from build123d import *

# Parameters (mm, degrees)
SCHIZZO1_R                   = 2.1
ESTRUSIONE_ESTRUSIONE1_DEPTH = 4
SCHIZZO2_R                   = 2.5
TAGLIO_ESTRUSIONE1_DEPTH     = 4
SCHIZZO3_R                   = 1.5
TAGLIO_ESTRUSIONE3_DEPTH     = 4


with BuildPart() as part:
    # Schizzo1 → Estrusione-Estrusione1 (new body)
    with BuildSketch(Plane.XY):
        with BuildLine():
            Line((69.543022759, -257.170330876), (65.21289574, -264.670330876))
            ThreePointArc((65.21289574, -264.670330876), (57.892387664, -271.990838952), (47.892387664, -274.670330876))
            Line((47.892387664, -274.670330876), (20.986398432, -274.670330876))
            ThreePointArc((20.986398432, -274.670330876), (10.986398432, -271.990838952), (3.665890356, -264.670330876))
            Line((3.665890356, -264.670330876), (-0.664236663, -257.170330876))
            Line((-0.664236663, -257.170330876), (-250.664236663, 175.842371016))
            Line((-250.664236663, 175.842371016), (-254.994363682, 183.342371016))
            ThreePointArc((-254.994363682, 183.342371016), (-257.673855606, 193.342371016), (-254.994363682, 203.342371016))
            Line((-254.994363682, 203.342371016), (-241.541369065, 226.643641206))
            ThreePointArc((-241.541369065, 226.643641206), (-234.22086099, 233.964149281), (-224.22086099, 236.643641206))
            Line((-224.22086099, 236.643641206), (-215.560606952, 236.643641206))
            Line((-215.560606952, 236.643641206), (284.439393048, 236.643641206))
            Line((284.439393048, 236.643641206), (293.099647086, 236.643641206))
            ThreePointArc((293.099647086, 236.643641206), (303.099647086, 233.964149281), (310.420155162, 226.643641206))
            Line((310.420155162, 226.643641206), (323.873149778, 203.342371016))
            ThreePointArc((323.873149778, 203.342371016), (326.552641702, 193.342371016), (323.873149778, 183.342371016))
            Line((323.873149778, 183.342371016), (319.543022759, 175.842371016))
            Line((319.543022759, 175.842371016), (69.543022759, -257.170330876))
        make_face()
        with Locations((34.439393048, -259.670330876)):
            Circle(SCHIZZO1_R, mode=Mode.SUBTRACT)
        with Locations((304.156271413, 207.493006111)):
            Circle(SCHIZZO1_R, mode=Mode.SUBTRACT)
        with Locations((-235.277485317, 207.493006111)):
            Circle(SCHIZZO1_R, mode=Mode.SUBTRACT)
    extrude(amount=ESTRUSIONE_ESTRUSIONE1_DEPTH)

    # Schizzo2 → Taglio-Estrusione1 (cut)
    with BuildSketch(Plane.XY.offset(4)):
        with Locations((34.439393048, 226.643641206)):
            Circle(SCHIZZO2_R)
        with Locations((-235.277485317, 207.493006111)):
            Circle(SCHIZZO2_R)
        with Locations((304.156271413, 207.493006111)):
            Circle(SCHIZZO2_R)
        with Locations((34.439393048, -259.670330876)):
            Circle(SCHIZZO2_R)
        with Locations((185.882768721, -35.66397993)):
            Circle(SCHIZZO2_R)
        with Locations((-117.003982625, -35.66397993)):
            Circle(SCHIZZO2_R)
    extrude(amount=-TAGLIO_ESTRUSIONE1_DEPTH, mode=Mode.SUBTRACT)

    # Schizzo3 → Taglio-Estrusione3 (cut)
    with BuildSketch(Plane.XY.offset(4)):
        with Locations((-47.560606952, 107.143641206)):
            Circle(SCHIZZO3_R)
        with Locations((70.439393048, 107.143641206)):
            Circle(SCHIZZO3_R)
        with Locations(Location((-47.560606952, 188.643641206, 0), (0, 0, 180))):
            Circle(SCHIZZO3_R)
        with Locations(Location((70.439393048, 188.643641206, 0), (0, 0, 180))):
            Circle(SCHIZZO3_R)
    extrude(amount=-TAGLIO_ESTRUSIONE3_DEPTH, mode=Mode.SUBTRACT)


solid = part.part
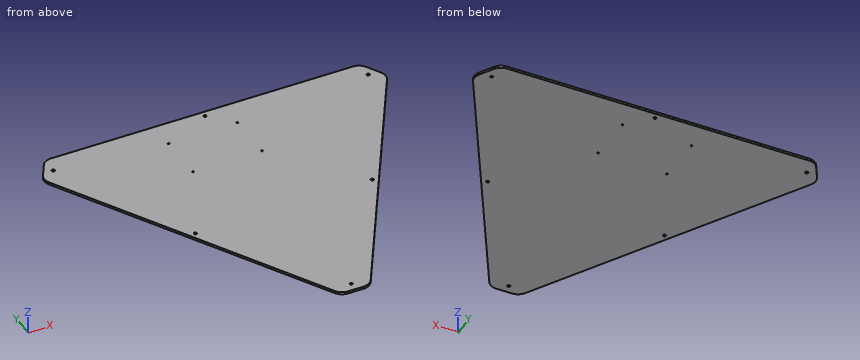
Build history of the part. All positions in model axes, mm. Give positions to 0.01 mm unless a question says otherwise; leave off trailing zeros. Write each loop counter-clockwise with the first axis right and the second up, starting at its lowest first coordinate (ties: lowest second). Pieces come first, ordered by that corner, then holes. Notation, with made-up numbers: (81, 18) - (85, 18) arc R20 cw to (85, 38) - close; hole circle Ø11 at (-15, 88). An arc over 180 degrees is marked (long way). Use one line per item in the form item = value. Start each with the question number.
1. Band-saw the part on A-A on z = 2.3. Count the separate pieces of the cut face and the enclosed holes in it, plus the area to 3 significant figures.
2. Band-saw the part on B-B on x = -209. Write the cut outline in (y, z), plus the area to 3 significant figures.
3. Band-saw the part on C-C on y = -80.5. Write the cut outline in (x, z), plus the area to 3 significant figures.
4. Drop flat-ended pins along their axis: pin 1 Ø1.5 at (y, z) = (148, 1) entering from +X; pin 2 Ø1.5 at (y, z) = (143.5, 3.5) entering from -X; pin 3 Ø1 at (y, z) = (137.5, 1.5) entering from -X. Give the stop position or say it passes through.
5. Probe line 1 (Y direction, x = 35, z = 3.3); line 2 (Y direction, x = -47, z = 2.1); line 3 (Y direction, x = 49, z = 3.45). List the from-to ranges inside material, lowest first. Write a range as [from, to].
Conclusion:
q1.separate_pieces = 1
q1.enclosed_holes = 10
q1.area = 174,000 mm²
q2.outline = (103.68, 0) - (236.64, 0) - (236.64, 4) - (103.68, 4) - close
q2.area = 532 mm²
q3.outline = (-102.66, 0) - (171.54, 0) - (171.54, 4) - (-102.66, 4) - close
q3.area = 1,100 mm²
q4.pin_1 = 303.9
q4.pin_2 = -232.42
q4.pin_3 = -228.82
q5.line_1 = [-274.67, -262.11], [-257.23, 224.21], [229.08, 236.64]
q5.line_2 = [-176.91, 105.75], [108.53, 187.25], [190.03, 236.64]
q5.line_3 = [-274.64, 236.64]
